from build123d import *

# Parameters (mm, degrees)
FILLET_1_R = 0.5


with BuildPart() as part:
    # 草图1 → 旋转1 (revolve)
    with BuildSketch(Plane(origin=(0, 0, 0), x_dir=(1, 0, 0), z_dir=(0, 1, 0)), mode=Mode.PRIVATE) as revolve_1_sk:
        Polygon((-140, 0), (-120, 11), (-80, 11), (-80, 13.95), (-1, 10), (-1, 9), (0, 9), (0, 0), align=None)
    revolve(revolve_1_sk.sketch.rotate(Axis((-857.450785528, 0, 0), (1, 0, 0)), 180), axis=Axis((-857.450785528, 0, 0), (1, 0, 0)))

    # 圆角1
    fillet_1_edges = [part.edges().sort_by_distance(p)[0] for p in [
        (0, 0, -9),
        (-1, 0, -9),
        (-80, 0, -11),
    ]]
    fillet(fillet_1_edges, radius=FILLET_1_R - 0.0001)  # a hair under: the kernel refuses the full size


solid = part.part
Model file for the job. Use its own axes, mm. A direction names the side the tool comes from. Give positions to 0.01 mm unless a question says otherwise; leave off trailing zeros. Order: outer loops, then holes, each group sorted by start corner. A loop starts at its lowest first (then second) coordinate and runs counter-clockwise, first axis right, second up. Notation, with made-up numbers: M 4,73.5 L 19,73.5 A32 ccw 19,108.5 Z; hole C -16,-31.5 d9. An arc over 180 degrees is marked long. Write item = value, one per line.
Q1. Tool access for faces 1 (the flat face through (0, 0, 0)), 2 (the flat face through (-1, 4, 9)), 3 (the flat face through (-80, -11.4, -3)): list every direction of +Z, -Z, +X, -X, +Y, -Y with a clear straight run to the whole face (end or side of a thin tool).
Derived:
face_1 = +Z, -Z, +X, +Y, -Y
face_2 = +X
face_3 = -X
Q2. Cut at A-A, the plane x = -77. List the corners of the cut face in (y, z), then the cut area to 3 significant figures.
Derived:
outline = C 0,0 d27.6
area = 598 mm2
Q3. Flat gauge pins, fed straight in: pin 1 (10 mm diameter, centred on y = 2, z = -9.5, fed in from +X); pin 2 (1 mm diameter, centred on x = -27.5, z = -6, fed in from +Y); pin 3 (6 mm diameter, centred on x = -94.5, z = 4, fed in from -Y); pin 4 (12 mm diameter, centred on y = -6, z = 5, fed in from -X). Where does each tip first touch, or does it go through?
Derived:
pin_1 = 0
pin_2 = 9.9
pin_3 = -10.95
pin_4 = -136.71
Q4. Drill centre lines: line 1 (Z direction, x = -86.5, y = 0.25); line 2 (Z direction, x = -71.5, y = -10.5) (3 decimals); line 3 (Y direction, x = -104.5, z = 0.5). Where is each one in solid material? Low to high. Write a range as [from, to].
Derived:
line_1 = [-11, 11]
line_2 = [-8.525, 8.525]
line_3 = [-10.99, 10.99]
Q5. Cut at B-B, the plane x = -93. List the corners of the cut face in (y, z).
Derived:
outline = C 0,0 d22
